Source: CAD feature listing. Evaluate the final solid. Frame: model axes, mm. A direction names the side the tool comes from. Coordinates: 2 decimals unless noted, no trailing zeros. Write each loop counter-clockwise with the first axis right and the second up, starting at its lowest first coordinate (ties: lowest second). Pieces come first, ordered by that corner, then holes. Notation, with made-up numbers: M 33,87.25 L 70,87.25 A12 ccw 70,91.25 Z; hole C 7,-15 d3. An arc over 180 degrees is marked long. Write item = value, one per line. Start each with the question number.
1. Section query C-C (z = -25). Output: boundary loops of the cut face in (x, y), then the cut area to 3 significant figures.
2. Pin query (flat end, axial travel): pin 1 Ø6 at (x, z) = (18, 1) entering from +Y; pin 2 Ø8 at (y, z) = (20.5, -9.5) entering from +X; pin 3 Ø0.7 at (x, y) = (9, 33.5) entering from -Z; pin 4 Ø10 at (x, z) = (2, 24.5) entering from +Y. Return the tip coordinate at first contact, or that it passes through.
3. Section query D-D (x = 2.25). Output: boundary loops of the cut face in (y, z).
4. Line query: line 1 along Z through (x, y) = (13, 20.75); line 2 along Y through (x, z) = (12.5, 23); line 3 along Z through (x, y) = (10.5, 32.5). Output: solid intervals per line, ascending.
5. Section query B-B (x = 14.5). Output: boundary loops of the cut face in (y, z).
6. Pull-direction query (Z, two-part tool) for faces 4 (the face through (10, 19, 33.97)), 5 (the face through (3.77, 29.95, 27.97)), 6 (the face through (9.86, 30.08, -29.31)); classes: pulls with the +Z half, pulls with the -Z half, needs draft (parallel to the pull), parting line crosses it, or undercut.
7. Access query for faces 1 (the face through (10, 20, 31.97)), 2 (the face through (13.45, 29.24, 28.69)), 3 (the face through (10, 33, 23.97)). Directions: +Z, -Z, +X, -X, +Y, -Y. A direction counts if a zero-diameter tool reaches every point of the face in a straight line with its end or side. Return the directions, or none.
8. Section query A-A (y = 18.5). Output: boundary loops of the cut face in (x, z).
```python
from build123d import *

# Parameters (mm, degrees)
BOSS_EXTRU_1_DEPTH         = 20
D_GAGEMENT_START           = 39.969957368
D_GAGEMENT_M2_51_OUTLINE_R = 1.55
D_GAGEMENT_M2_51_DEPTH     = 2.030042632


# Read off the part's stored shape, not the designer's step: Dégagement M2.51
with BuildPart() as part:
    # Esquisse1 → Boss.-Extru.1 (new body)
    with BuildSketch(Plane(origin=(0, 0, 0), x_dir=(0, 0, -1), z_dir=(1, 0, 0))):
        with BuildLine():
            Line((-31.97, 24.039948003), (-31.97, 15.66))
            Line((-31.97, 15.66), (31.97, 15.66))
            Line((31.97, 15.66), (31.97, 24.039948003))
            ThreePointArc((31.97, 24.039948003), (28.253337793, 28.315170908), (23.97, 32.022478043))
            Line((23.97, 32.022478043), (23.97, 34.488245824))
            ThreePointArc((23.97, 34.488245824), (29.380578316, 30.013024137), (33.97, 24.698969614))
            Line((33.97, 24.698969614), (33.97, 13.66))
            Line((33.97, 13.66), (-33.97, 13.66))
            Line((-33.97, 13.66), (-33.97, 24.698969614))
            ThreePointArc((-33.97, 24.698969614), (-29.380578316, 30.013024137), (-23.97, 34.488245824))
            Line((-23.97, 34.488245824), (-23.97, 32.022478043))
            ThreePointArc((-23.97, 32.022478043), (-28.253337793, 28.315170908), (-31.97, 24.039948003))
        make_face()
    extrude(amount=BOSS_EXTRU_1_DEPTH)

    # Dégagement M2.51 outline → Dégagement M2.51 (cut)
    with BuildSketch(Plane(origin=(0, 0, 0), x_dir=(1, 0, 0), z_dir=(0, 0.7149556691384648, -0.6991697870809138)).offset(D_GAGEMENT_START)):
        with Locations((5, 0)):
            Circle(D_GAGEMENT_M2_51_OUTLINE_R)
        with Locations((15, 0)):
            Circle(D_GAGEMENT_M2_51_OUTLINE_R)
    d_gagement_m2_51 = extrude(amount=D_GAGEMENT_M2_51_DEPTH, mode=Mode.SUBTRACT)

    # Symétrie1: Dégagement M2.51 across plane
    add(d_gagement_m2_51.mirror(Plane.XY), mode=Mode.SUBTRACT)


solid = part.part
```
Results are:
q1.outline = M 0,13.66 L 20,13.66 L 20,15.66 L 0,15.66 Z; M 0,31.22 L 20,31.22 L 20,33.75 L 0,33.75 Z
q1.area = 90.5 mm^2
q2.pin_1 = 15.66
q2.pin_2 = through
q2.pin_3 = -25.79
q2.pin_4 = 34.49
q3.outline = M 13.66,-33.97 L 24.7,-33.97 A42 ccw 34.49,-23.97 L 32.02,-23.97 A40 cw 24.04,-31.97 L 15.66,-31.97 L 15.66,31.97 L 24.04,31.97 A40 cw 32.02,23.97 L 34.49,23.97 A42 ccw 24.7,33.97 L 13.66,33.97 Z
q4.line_1 = -33.97 to -31.97, 31.97 to 33.97
q4.line_2 = 13.66 to 15.66
q4.line_3 = -26.6 to -23.97, 23.97 to 26.6
q5.outline = M 13.66,-33.97 L 24.7,-33.97 A42 ccw 28.98,-30.4 L 27.55,-29 A40 cw 24.04,-31.97 L 15.66,-31.97 L 15.66,31.97 L 24.04,31.97 A40 cw 27.55,29 L 28.98,30.4 A42 ccw 24.7,33.97 L 13.66,33.97 Z; M 29.6,-26.9 L 31.04,-28.3 A42 ccw 34.49,-23.97 L 32.02,-23.97 A40 cw Z; M 29.6,26.9 A40 cw 32.02,23.97 L 34.49,23.97 A42 ccw 31.04,28.3 Z
q6.face_4 = pulls with the +Z half
q6.face_5 = undercut
q6.face_6 = pulls with the -Z half
q7.face_1 = +X, -X
q7.face_2 = none
q7.face_3 = +X, -X, +Y
q8.outline = M 0,-33.97 L 20,-33.97 L 20,-31.97 L 0,-31.97 Z; M 0,31.97 L 20,31.97 L 20,33.97 L 0,33.97 Z
